Verification items for the finished model (mm, model axes). Round coordinates to 2 decimals unless told otherwise and drop trailing zeros. Loops run counter-clockwise (first coordinate to the right, second up) from the corner with the lowest first, then second, coordinate; pieces in that order, holes last. Notation, with made-up numbers: (-34.5, 89) -> (14.5, 89) arc R18 cw to (14.5, 93) -> close; hole circle Ø6 at (53.5, -20). An arc over 180 degrees is marked (long way). Use CSV: the item, a comma, the result in double quotes. Start each with the question number.
Autodesk Inventor part; units mm, degrees
ref_plane "YZ Plane" through (0, 0, 0) normal (1, 0, 0) x (0, 1, 0)
ref_plane "XZ Plane" through (0, 0, 0) normal (0, 1, 0) x (-1, 0, 0)
ref_plane "XY Plane" through (0, 0, 0) normal (0, 0, 1) x (1, 0, 0)
sketch "Sketch1" plane through (0, 0, 0) normal (0, 1, 0) x (-1, 0, 0)
  line L0 (0, 0) -> (16, 0)
  line L1 (16, 0) -> (16, -2)
  line L2 (16, -2) -> (0, -2)
  line L3 (0, -2) -> (0, 0)
  line L4 (16, -1) -> (15, -1)
  line L5 (8, -2) -> (8, -1)
  circle A0 centre (15, -1) radius 0.5
  circle A1 centre (1, -1) radius 0.5
  dimension "d0" = 16
  dimension "d1" = 2
  dimension "d2" = 1
  dimension "d3" = 1
extrude "Extrusion1" add sketch "Sketch1" along normal blind 2
properties part number "short_link_v1"
Q1. Cross-section at A-A (x = -15). Record the boundary of the cut face in (y, z), and give its area (3 significant figures).
Q2. Release check for a two-part mould opening along Z. For faces 1 (the face through (-16, 1, -1)), 2 (the face through (-8, 1, 0)), 3 (the face through (-0.6, 1, -0.7)) record: +Z half, -Z half, draft (parallel to the pull), parting line (faces both ways), or undercut.
Q3. Cross-section at C-C (y = 0.35). Record the boundary of the cut face in (x, z), and give its area (3 significant figures).
Q4. Cross-section at B-B (z = -1). Record the boundary of the cut face in (x, y).
Q5. Thickness scan on L1, parallel to X at y = 1.1, z = -0.95; L2, parallel to Z at x = -15, y = 0.65; L3, parallel to X at y = 0.4, z = -0.7. Record the ranges inside material, lowest first. Write a range as from..to.
Answer list:
1,outline,"(0, -2) -> (2, -2) -> (2, -1.5) -> (0, -1.5) -> close; (0, -0.5) -> (2, -0.5) -> (2, 0) -> (0, 0) -> close"
1,area,"2.00 mm2"
2,face 1,"draft"
2,face 2,"+Z half"
2,face 3,"undercut"
3,outline,"(-16, -2) -> (0, -2) -> (0, 0) -> (-16, 0) -> close; hole circle Ø1 at (-15, -1); hole circle Ø1 at (-1, -1)"
3,area,"30.4 mm2"
4,outline,"(-16, 0) -> (-15.5, 0) -> (-15.5, 2) -> (-16, 2) -> close; (-14.5, 0) -> (-1.5, 0) -> (-1.5, 2) -> (-14.5, 2) -> close; (-0.5, 0) -> (0, 0) -> (0, 2) -> (-0.5, 2) -> close"
5,L1,"x = -16..-15.5, -14.5..-1.5, -0.5..0"
5,L2,"z = -2..-1.5, -0.5..0"
5,L3,"x = -16..-15.4, -14.6..-1.4, -0.6..0"
